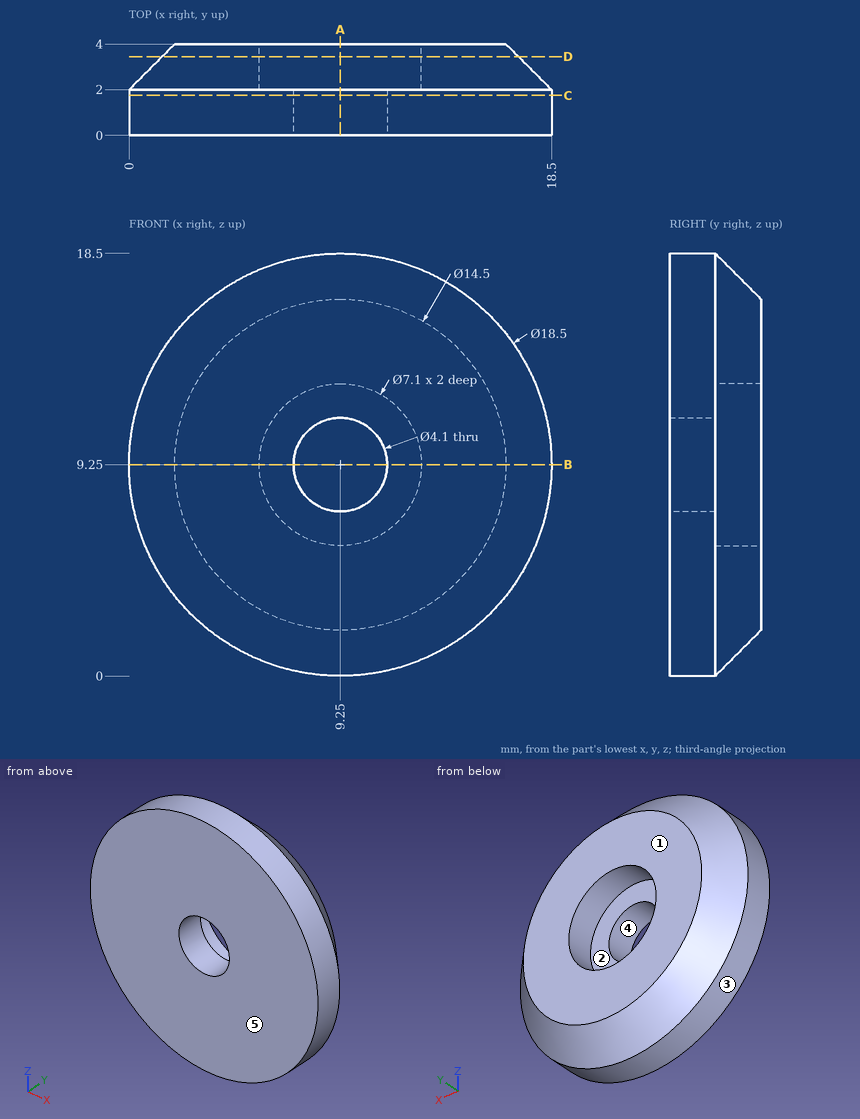
Check sheet for the drawn part. Datum: minimum x, y, z corner. Units: mm. A direction names the side the tool comes from. Give positions to 0.01 mm unless a question says otherwise; leave off trailing zeros. Write each loop counter-clockwise with the first axis right and the second up, starting at its lowest first coordinate (ties: lowest second). Pieces come first, ordered by that corner, then holes. Notation, with made-up numbers: (30, 21) -> (62, 21) arc R9 cw to (62, 32) -> close; hole circle Ø8 at (34.25, -6.75). An arc over 180 degrees is marked (long way). Use one line per item in the form item = value. Start each with the question number.
1. Section check C-C (y = 1.75). Record the cut outline in (x, z).
2. Access from +Z, -Z, +X, -X, +Y, -Y to the whole of each face (thin tool, end or side, straight path). Record for the marked faces 1 and 2.
3. Thickness scan on line 1 along X through (y, z) = (1.55, 9.25); line 2 along Y through (x, z) = (7.25, 11.75); line 3 along X through (y, z) = (2.4, 9.75). Record the ranges inside material, lowest first. Write a range as from..to.
4. Mould release check, pull along Z, two halves, no side actions. Record for the marked faces 3, 4 and 5: pulls with the +Z half, pulls with the -Z half, needs draft (parallel to the pull), parting line crosses it, or undercut.
5. Section check A-A (x = 9.25). Record the cut outline in (y, z).
6. Section check B-B (z = 9.25). Record the cut outline in (x, y), and give its area (3 significant figures).
7. Go/stop test with flat-tipped pins: P1, Ø2, axis at x = 10.5, z = 8, coming from the +Y side; P2, Ø1, axis at x = 14, y = 3, coming from the +Z side; P3, Ø1.5, axis at y = 0.5, z = 3, coming from the -X side. Record where each tip stops, or that it passes through.
8. Section check D-D (y = 3.45). Record the cut outline in (x, z), and give its area (3 significant figures).
Conclusion:
q1.outline = circle Ø18.5 at (9.25, 9.25); hole circle Ø4.1 at (9.25, 9.25)
q2.face_1 = +Z, -Z, +X, -X, +Y
q2.face_2 = +Y
q3.line_1 = 0..7.2, 11.3..18.5
q3.line_2 = 0..2
q3.line_3 = 0.41..5.74, 12.76..18.09
q4.face_3 = parting line crosses it
q4.face_4 = undercut
q4.face_5 = needs draft
q5.outline = (0, 0) -> (2, 0) -> (4, 2) -> (4, 5.7) -> (2, 5.7) -> (2, 7.2) -> (0, 7.2) -> close; (0, 11.3) -> (2, 11.3) -> (2, 12.8) -> (4, 12.8) -> (4, 16.5) -> (2, 18.5) -> (0, 18.5) -> close
q6.outline = (0, 0) -> (7.2, 0) -> (7.2, 2) -> (5.7, 2) -> (5.7, 4) -> (2, 4) -> (0, 2) -> close; (11.3, 0) -> (18.5, 0) -> (18.5, 2) -> (16.5, 4) -> (12.8, 4) -> (12.8, 2) -> (11.3, 2) -> close
q6.area = 47.6 mm²
q7.P1 = 2
q7.P2 = 16.68
q7.P3 = 1.81
q8.outline = circle Ø15.6 at (9.25, 9.25); hole circle Ø7.1 at (9.25, 9.25)
q8.area = 152 mm²
